Could you check a few things on this model? Use its own coordinates, in mm. Give positions to 0.01 mm unless a question says otherwise; leave off trailing zeros. Order: outer loops, then holes, each group sorted by start corner. A loop starts at its lowest first (then second) coordinate and runs counter-clockwise, first axis right, second up. Notation, with made-up numbers: (-1, -1) -> (36, -1) arc R25 cw to (36, 21) -> close; hole circle Ø3 at (-23, 85.25). An arc over 180 degrees is marked (long way). Answer as CSV lines item,"result". Start each with the question number.
(1) I want a section at B-B (x = -38.5). Please give me the cut outline in (y, z) (3 decimals).
(2) I want a section at A-A (z = 0.1). Please give me the cut outline in (x, y).
(3) I want a section at C-C (x = 42.5). Please give me the cut outline in (y, z) (3 decimals), plus the area to 3 significant figures.
(4) I need wall thicknesses on L1, parallel to X at y = -32, z = 0.1; L2, parallel to X at y = 40, z = 0.55; L3, parallel to Y at x = -38.5, z = 0.2. Which ranges of each line are inside material? Lowest first, please.
```python
from build123d import *

# Parameters (mm, degrees)
F1_DEPTH = 0.635


with BuildPart() as f1:
    # F0 (on Top) → F1 (new body, symmetric)
    with BuildSketch(Plane.XY):
        with BuildLine():
            Line((-31.75, -50.8), (31.75, -50.8))
            ThreePointArc((31.75, -50.8), (45.220384, -45.220384), (50.8, -31.75))
            Line((50.8, -31.75), (50.8, 31.75))
            ThreePointArc((50.8, 31.75), (45.220384, 45.220384), (31.75, 50.8))
            Line((31.75, 50.8), (-31.75, 50.8))
            ThreePointArc((-31.75, 50.8), (-45.220384, 45.220384), (-50.8, 31.75))
            Line((-50.8, 31.75), (-50.8, -31.75))
            ThreePointArc((-50.8, -31.75), (-45.220384, -45.220384), (-31.75, -50.8))
        make_face()
    extrude(amount=F1_DEPTH, both=True)


solid = f1.part
```
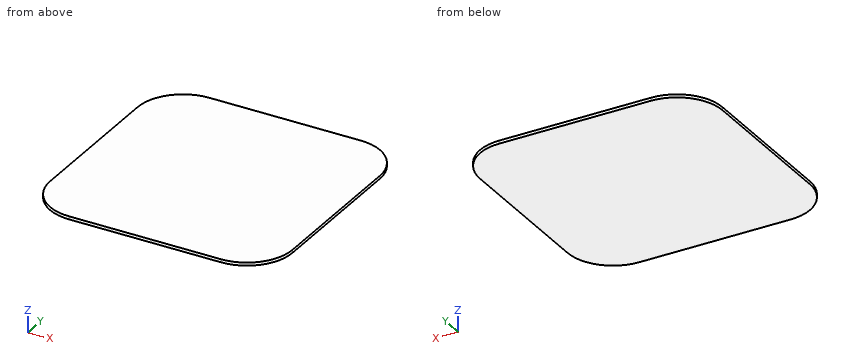
Final values:
1,outline,"(-49.564, -0.635) -> (49.564, -0.635) -> (49.564, 0.635) -> (-49.564, 0.635) -> close"
2,outline,"(-50.8, -31.75) arc R19.05 ccw to (-31.75, -50.8) -> (31.75, -50.8) arc R19.05 ccw to (50.8, -31.75) -> (50.8, 31.75) arc R19.05 ccw to (31.75, 50.8) -> (-31.75, 50.8) arc R19.05 ccw to (-50.8, 31.75) -> close"
3,outline,"(-47.477, -0.635) -> (47.477, -0.635) -> (47.477, 0.635) -> (-47.477, 0.635) -> close"
3,area,"121 mm²"
4,L1,"-50.8 to 50.8"
4,L2,"-48.92 to 48.92"
4,L3,"-49.56 to 49.56"
